from build123d import *

# Parameters (mm, degrees)
RUNROUTE_R           = 16.75
RUNEXTRUDE_DEPTH     = 35
OUTLETROUTE_R        = 16.75
OUTLETEXTRUDE_DEPTH  = 35
TEESHELL_START       = -35
TEESHELL_OUTLINE_R   = 12.25
TEESHELL_DEPTH       = 70
TEESHELL_START_2     = -1e-07
TEESHELL_2_OUTLINE_R = 12.25
TEESHELL_2_DEPTH     = 35.0000001
TEECHAMFER_SIZE      = 1


with BuildPart() as part:
    # RunRoute → RunExtrude (new body)
    with BuildSketch(Plane(origin=(0, 0, 0), x_dir=(0, 0, -1), z_dir=(1, 0, 0))):
        Circle(RUNROUTE_R)
    runextrude = extrude(amount=RUNEXTRUDE_DEPTH)

    # RunExtrudeMirror: RunExtrude across plane
    add(runextrude.mirror(Plane(origin=(0, 0, 0), x_dir=(0, 0, 1), z_dir=(1, 0, 0))))

    # OutletRoute → OutletExtrude (add)
    with BuildSketch(Plane(origin=(0, 0, 0), x_dir=(1, 0, 0), z_dir=(0, 1, 0))):
        with Locations(Location((0, 0, 0), (0, 0, 270))):
            Circle(OUTLETROUTE_R)
    extrude(amount=OUTLETEXTRUDE_DEPTH)

    # TeeShell: read off the stored shape, not the designer's step
    # TeeShell outline → TeeShell (cut)
    with BuildSketch(Plane.YZ.offset(TEESHELL_START)):
        Circle(TEESHELL_OUTLINE_R)
    extrude(amount=TEESHELL_DEPTH, mode=Mode.SUBTRACT)

    # TeeShell 2 outline → TeeShell 2 (cut)
    with BuildSketch(Plane(origin=(0, 0, 0), x_dir=(1, 0, 0), z_dir=(0, 1, 0)).offset(TEESHELL_START_2)):
        Circle(TEESHELL_2_OUTLINE_R)
    extrude(amount=TEESHELL_2_DEPTH, mode=Mode.SUBTRACT)

    # TeeChamfer
    # the kernel refuses this chamfer: 1 mm, written as the material it takes off along each edge
    with BuildSketch(Plane(origin=(0, 35, 0), x_dir=(0, 0, 1), z_dir=(-1, 0, 0))) as teechamfer_piece_1:
        Polygon((16.75, -TEECHAMFER_SIZE), (16.75 - TEECHAMFER_SIZE, 0), (16.75, 0), align=None)
    revolve(axis=Axis((0, 35, 0), (0, 1, 0)), mode=Mode.SUBTRACT)
    with BuildSketch(Plane(origin=(35, 0, 0), x_dir=(0, 0, -1), z_dir=(0, -1, 0))) as teechamfer_piece_2:
        Polygon((16.75, -TEECHAMFER_SIZE), (16.75 - TEECHAMFER_SIZE, 0), (16.75, 0), align=None)
    revolve(axis=Axis((35, 0, 0), (1, 0, 0)), mode=Mode.SUBTRACT)
    with BuildSketch(Plane(origin=(-35, 0, 0), x_dir=(0, 0, -1), z_dir=(0, -1, 0))) as teechamfer_piece_3:
        Polygon((16.75, TEECHAMFER_SIZE), (16.75 - TEECHAMFER_SIZE, 0), (16.75, 0), align=None)
    revolve(axis=Axis((-35, 0, 0), (1, 0, 0)), mode=Mode.SUBTRACT)


solid = part.part
The listing builds one solid part. Answer for the finished solid, in the listing's coordinates (mm). A direction names the side the tool comes from. Round coordinates to 2 decimals unless told otherwise and drop trailing zeros. Write each loop counter-clockwise with the first axis right and the second up, starting at its lowest first coordinate (ties: lowest second). Pieces come first, ordered by that corner, then holes. Notation, with made-up numbers: (82, -8) - (103, -8) arc R33 ccw to (103, 23) - close; hole circle Ø4 at (23, -13). An arc over 180 degrees is marked (long way). Use a Markdown table: item, result. Add a question column.
1. Consider line 1 (Z direction, x = 19, y = 0); line 2 (X direction, y = 13, z = 0). Determine where each line is inside the solid, lowest interval first.
2. The part is cut by section A-A (z = 0). Write down the section's boundary in (x, y), and give its area (3 significant figures).
3. The part is cut by section C-C (y = 26). Write down the section's boundary in (x, z), and give its area (3 significant figures).
4. Flat-ended cylindrical pins translate along their axes: P1, Ø6, axis at x = -25.5, y = -10.5, coming from the -Z side; P2, Ø14.5, axis at x = 0, z = 0, coming from the +Y side; P3, Ø2, axis at x = 21.5, z = -5, coming from the +Y side. Find the tip coordinate at first contact, or state that the pin passes through.
5. For a pull along X with two mould halves and no side action, classify faces 3 (the face through (-35, -8.1, 9.4)), 4 (the face through (-1.595, 21.144, -12.146)), 5 (the face through (11.32, 20.54, -12.345)) as +X half, -X half, draft (parallel to the pull), parting line (faces both ways), or undercut.
6. A tool of negligible diameter and unlimited length cuts with its end or side. For faces 1 (the face through (35, -8.1, 9.4)), 2 (the face through (0.48, -14.86, -7.73)), from which of +Z, -Z, +X, -X, +Y, -Y can it reach the whole face along a straight path? Write none if from no direction.
7. The part is cut by section B-B (x = 0). Write down the section's boundary in (y, z), and give its area (3 significant figures).
Reported:
| question | item | result |
|---|---|---|
| 1 | line 1 | -16.75 to -12.25, 12.25 to 16.75 |
| 1 | line 2 | -35 to -12.25, 12.25 to 35 |
| 2 | outline | (-35, -15.75) - (-34, -16.75) - (34, -16.75) - (35, -15.75) - (35, -12.25) - (-35, -12.25) - close; (-35, 12.25) - (-12.25, 12.25) - (-12.25, 35) - (-15.75, 35) - (-16.75, 34) - (-16.75, 16.75) - (-34, 16.75) - (-35, 15.75) - close; (12.25, 12.25) - (35, 12.25) - (35, 15.75) - (34, 16.75) - (16.75, 16.75) - (16.75, 34) - (15.75, 35) - (12.25, 35) - close |
| 2 | area | 681 mm^2 |
| 3 | outline | circle Ø33.5 at (0, 0); hole circle Ø24.5 at (0, 0) |
| 3 | area | 410 mm^2 |
| 4 | P1 | z = -14.98 |
| 4 | P2 | y = -9.87 |
| 4 | P3 | y = 16.27 |
| 5 | face 3 | -X half |
| 5 | face 4 | undercut |
| 5 | face 5 | parting line |
| 6 | face 1 | +Z, -Z, +X, +Y, -Y |
| 6 | face 2 | none |
| 7 | outline | (0, -16.75) - (34, -16.75) - (35, -15.75) - (35, -12.25) - (0, -12.25) arc R12.25 cw to (0, 12.25) - (35, 12.25) - (35, 15.75) - (34, 16.75) - (0, 16.75) arc R16.75 ccw to start |
| 7 | area | 519 mm^2 |
